```python
from build123d import *

# Parameters (mm, degrees)
BOSS_EXTRUDE1_DEPTH = 1
BOSS_EXTRUDE2_START = -1.5
BOSS_EXTRUDE2_DEPTH = 3
CIRPATTERN1_COUNT   = 3
CIRPATTERN1_ANGLE   = 180


# Read off the part's stored shape, not the designer's step: Boss-Extrude2
with BuildPart() as part:
    # Sketch1 → Boss-Extrude1 (new body)
    with BuildSketch(Plane.XY):
        Polygon((13, -9.565), (13, 9.565), (-13, 9.565), (-13, -9.565), (-19, -9.565), (-19, -41.315), (-13, -41.315), (-13, -15.315), (13, -15.315), (13, -41.315), (19, -41.315), (19, -9.565), align=None)
    extrude(amount=BOSS_EXTRUDE1_DEPTH)

    # Boss-Extrude2 outline → Boss-Extrude2 (add)
    with BuildSketch(Plane(origin=(0, -28.315, 0), x_dir=(-1, 0, 0), z_dir=(0, -1, 0)).offset(BOSS_EXTRUDE2_START)):
        with BuildLine():
            Line((-11.23522271, -2.644286359), (-11.23522271, -1.144286359))
            add(Edge.make_bspline(
                [(-11.23522271, -1.144286359), (-11.740174878, -0.757764956), (-12.028679887, -1.161534837), (-12.227869222, -1.503002268), (-12.747184273, -1.488774458), (-13, -1)],
                knots=[0, 0, 0, 0, 0, 0, 1, 1, 1, 1, 1, 1], degree=5))
            Line((-13, -1), (-14.5, -1))
            add(Edge.make_bspline(
                [(-14.5, -1), (-13.760887065, -2.414906572), (-12.67824158, -3.40768712), (-12.345095428, -2.525951835), (-11.7215069, -2.450856602), (-11.23522271, -2.644286359)],
                knots=[0, 0, 0, 0, 0, 0, 1, 1, 1, 1, 1, 1], degree=5))
        make_face()
    boss_extrude2 = extrude(amount=BOSS_EXTRUDE2_DEPTH)

    # CirPattern1: Boss-Extrude2 ×3 about axis
    cirpattern1_axis = Axis((0, -28.315, 1.05), (0, 0, 1))
    for i in range(1, CIRPATTERN1_COUNT):
        add(boss_extrude2.rotate(cirpattern1_axis, i * CIRPATTERN1_ANGLE / (CIRPATTERN1_COUNT - 1)))


solid = part.part
```
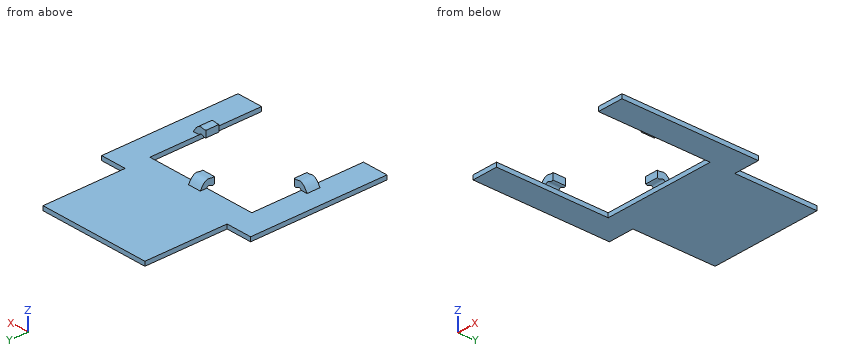
Could you check a few things on this model? Use its own coordinates, in mm. Give positions to 0.01 mm unless a question says otherwise; leave off trailing zeros. Order: outer loops, then holes, each group sorted by start corner. A loop starts at its lowest first (then second) coordinate and runs counter-clockwise, first axis right, second up.
Q1. Suppose I cut it at C-C, the plane x = -16. Write out the boundary of the cut face in (y, z) (3 decimals), and give its area (4 significant figures).
Q2. Suppose I cut it at A-A, the plane y = -25.5. Write out the boundary of the cut face in (x, z).
Q3. I'm going to push flat-ended pins straight in: P1, Ø1.1, axis at y = -2, z = 0.5, coming from the +X side; P2, Ø6, axis at x = 10.5, y = -14, coming from the +Z side; P3, Ø1.4, axis at y = -15.5, z = 2, coming from the -X side. Where does each tip first touch, or does it pass through?
Q4. If I drill on line 1 along X through (y, z) = (-35, 0.6); line 2 along Y through (x, z) = (-14.5, 0.3) (3 decimals); line 3 along Z through (x, y) = (17.5, -20), over which ranges is the centre line in solid material (lowest first)?
Q5. Suppose I cut it at D-D, the plane z = 1.9. Count the separate pieces of the cut face and the enclosed holes in it, and give its area (3 significant figures).
Q6. Suppose I cut it at B-B, the plane y = 1.5. Write out the boundary of the cut face in (x, z).
Solution:
1. outline: (-41.315, 0) - (-9.565, 0) - (-9.565, 1) - (-41.315, 1) - close
1. area: 31.75 mm2
2. outline: (-19, 0) - (-13, 0) - (-13, 1) - (-19, 1) - close; (13, 0) - (19, 0) - (19, 1) - (13, 1) - close
3. P1: stops at x = 13
3. P2: stops at z = 1
3. P3: stops at x = -1.5
4. line 1: x = -19 to -13, 13 to 19
4. line 2: y = -41.315 to -9.565
4. line 3: z = 0 to 1
5. separate pieces: 3
5. enclosed holes: 0
5. area: 24.2 mm2
6. outline: (-13, 0) - (13, 0) - (13, 1) - (-13, 1) - close
